from build123d import *

# Parameters (mm, degrees)
SKETCH1_R           = 25.4
SKETCH1_R_2         = 9.525
SKETCH1_R_3         = 4.7625
BOSS_EXTRUDE1_DEPTH = 15.875
SKETCH1_3_R         = 9.525
SKETCH1_3_R_2       = 4.7625
BOSS_EXTRUDE2_DEPTH = 9.525
FILLET1_R           = 2.54
BOSS_EXTRUDE3_DEPTH = 3.175


with BuildPart() as part:
    # Sketch1 → Boss-Extrude1 (new body)
    with BuildSketch(Plane.XY):
        Circle(SKETCH1_R)
        Circle(SKETCH1_R_2, mode=Mode.SUBTRACT)
        Circle(SKETCH1_R_2)
        Circle(SKETCH1_R_3, mode=Mode.SUBTRACT)
    extrude(amount=BOSS_EXTRUDE1_DEPTH)

    # Sketch1_3 → Boss-Extrude2 (add)
    with BuildSketch(Plane.XY):
        Circle(SKETCH1_3_R)
        Circle(SKETCH1_3_R_2, mode=Mode.SUBTRACT)
    extrude(amount=-BOSS_EXTRUDE2_DEPTH)

    # Fillet1
    fillet1_edges = [part.edges().sort_by_distance(p)[0] for p in [
        (-9.525, 0, 0),
    ]]
    fillet(fillet1_edges, radius=FILLET1_R)

    # Sketch2 → Boss-Extrude3 (add)
    with BuildSketch(Plane.XY.offset(15.875)):
        with BuildLine():
            Line((-1.27, 4.590044254), (-1.27, -4.590044254))
            ThreePointArc((-1.27, -4.590044254), (0, -4.7625), (1.27, -4.590044254))
            Line((1.27, -4.590044254), (1.27, 4.590044254))
            ThreePointArc((1.27, 4.590044254), (0, 4.7625), (-1.27, 4.590044254))
        make_face()
    extrude(amount=-BOSS_EXTRUDE3_DEPTH)


solid = part.part
The model under review builds one solid part; all positions refer to its coordinate system, in mm. A direction names the side the tool comes from. Coordinates: 2 decimals unless noted, no trailing zeros. Write each loop counter-clockwise with the first axis right and the second up, starting at its lowest first coordinate (ties: lowest second). Pieces come first, ordered by that corner, then holes. Notation, with made-up numbers: (50.5, 79.5) - (95.5, 79.5) arc R26 cw to (95.5, 100.5) - close; hole circle Ø8 at (-8, -2). An arc over 180 degrees is marked (long way). Answer as a JSON object with one key per item and string values. Group by question number.
1. Clearance check with flat-ended pins moving along their axes: pin 1 Ø1.6 at (y, z) = (-1, 14) entering from +X; pin 2 Ø10 at (x, z) = (16.5, 1) entering from +Y; pin 3 Ø2 at (y, z) = (13.5, -0.5) entering from -X. State where each tip first meets the part, or that it passes through.
2. Mouldability with a two-part tool opening along X and no side actions: class faces 4 (the face through (1.27, 0, 14)), 5 (the face through (0, 0, 15.875)), 6 (the face through (-7.559, -5.796, -5.984)) as pulls with the +X half, pulls with the -X half, needs draft (parallel to the pull), parting line crosses it, or undercut.
3. To check wall thickness, follow probe 1 along Y at (x, z) = (0, -4) (1 decimal); probe 2 along X at (y, z) = (-2.5, 13.5); probe 3 along Y at (x, z) = (0, 7.75). State the ranges of each line that lie inside material, in increasing order.
4. Add section C-C (x = 0). Give the boundary of the cut face in (y, z) (1 decimal).
5. Add section A-A (y = 0). Give the boundary of the cut face in (x, z) (1 decimal).
6. Machinability: for faces 1 (the face through (4.543, 1.431, 3.353)), 2 (the face through (-1.27, 0, 14)), 3 (the face through (-4.4, 2.3, -9.525)), which of the approach directions +Z, -Z, +X, -X, +Y, -Y give a long, thin tool a straight path to every point of the face, cutting with its end or side? Answer none if there is none.
7. Add section D-D (y = -14). Give the boundary of the cut face in (x, z) (3 decimals), plus the area to 3 significant figures.
Findings:
{
 "1": {"pin 1": "x = 25.4", "pin 2": "y = 22.65", "pin 3": "x = -22.04"},
 "2": {"face 4": "undercut", "face 5": "needs draft", "face 6": "parting line crosses it"},
 "3": {"probe 1": "-9.5 to -4.8, 4.8 to 9.5", "probe 2": "-25.28 to -4.05, -1.27 to 1.27, 4.05 to 25.28", "probe 3": "-25.4 to -4.76, 4.76 to 25.4"},
 "4": {"outline": "(-25.4, 0) - (-12.1, 0) arc R2.5 cw to (-9.5, -2.5) - (-9.5, -9.5) - (-4.8, -9.5) - (-4.8, 12.7) - (4.8, 12.7) - (4.8, -9.5) - (9.5, -9.5) - (9.5, -2.5) arc R2.5 cw to (12.1, 0) - (25.4, 0) - (25.4, 15.9) - (-25.4, 15.9) - close"},
 "5": {"outline": "(-25.4, 0) - (-12.1, 0) arc R2.5 cw to (-9.5, -2.5) - (-9.5, -9.5) - (-4.8, -9.5) - (-4.8, 15.9) - (-25.4, 15.9) - close; (-1.3, 12.7) - (1.3, 12.7) - (1.3, 15.9) - (-1.3, 15.9) - close; (4.8, -9.5) - (9.5, -9.5) - (9.5, -2.5) arc R2.5 cw to (12.1, 0) - (25.4, 0) - (25.4, 15.9) - (4.8, 15.9) - close"},
 "6": {"face 1": "-Z", "face 2": "+Z, -Z", "face 3": "-Z, +X, -X, +Y, -Y"},
 "7": {"outline": "(-21.193, 0) - (21.193, 0) - (21.193, 15.875) - (-21.193, 15.875) - close", "area": "673 mm²"}
}
